For this review, take the finished solid that the model builds, in its own axes (mm). Give positions to 0.01 mm unless a question says otherwise; leave off trailing zeros. Write each loop counter-clockwise with the first axis right and the second up, starting at its lowest first coordinate (ties: lowest second). Pieces come first, ordered by that corner, then holes.
1) We need section A-A on x = 132. Give the boundary of the cut face in (y, z).
2) We need section C-C on y = 2.05. Give the boundary of the cut face in (x, z) (1 decimal), and give its area (3 significant figures).
3) We need section B-B on z = 356.5. Give the boundary of the cut face in (x, y), and give its area (3 significant figures).
4) Wall thickness on line 1 along Z through (x, y) = (-104, 2.1); line 2 along Z through (x, y) = (-29, 1.95): over which ranges is each line inside the solid? List them lowest first.
5) For P1, Ø1.5, axis at y = 1, z = 304.5, coming from the -X side, flat-tipped, find the tip position at first contact; note if it passes through.
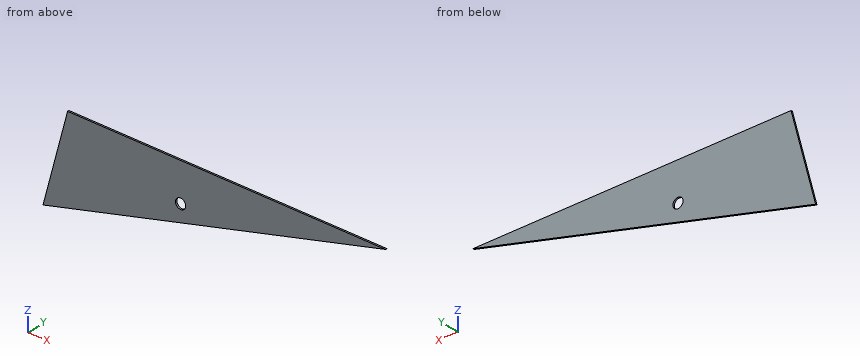
from build123d import *

# Parameters (mm, degrees)
BOSS_EXTRUDE1_DEPTH = 2.54
SKETCH2_R           = 7.9375
CUT_EXTRUDE1_DEPTH  = 2.54
CUT_EXTRUDE2_DEPTH  = 2.54


with BuildPart() as part:
    # Sketch1 → Boss-Extrude1 (new body)
    with BuildSketch(Plane(origin=(0, 0, 0), x_dir=(1, 0, 0), z_dir=(0, 1, 0))):
        Polygon((-288.635862607, -221.384099055), (-288.635862607, -365.420521122), (248.915382685, -365.420521122), align=None)
    extrude(amount=BOSS_EXTRUDE1_DEPTH)

    # Sketch2 → Cut-Extrude1 (cut)
    with BuildSketch(Plane(origin=(0, 2.54, 0), x_dir=(1, 0, 0), z_dir=(0, 1, 0))):
        with Locations((-72.735862607, -305.530344684)):
            Circle(SKETCH2_R)
    extrude(amount=-CUT_EXTRUDE1_DEPTH, mode=Mode.SUBTRACT)

    # Sketch3 → Cut-Extrude2 (cut)
    with BuildSketch(Plane.XZ):
        Polygon((-288.635862607, 221.384099055), (-250.041419634, 365.420521122), (-288.635862607, 365.420521122), align=None)
    extrude(amount=-CUT_EXTRUDE2_DEPTH, mode=Mode.SUBTRACT)


solid = part.part
Results list:
1. outline: (0, 334.09) - (2.54, 334.09) - (2.54, 365.42) - (0, 365.42) - close
2. outline: (-288.6, 221.4) - (248.9, 365.4) - (-250, 365.4) - close; hole circle Ø15.9 at (-72.7, 305.5)
2. area: 35,700 mm2
3. outline: (-252.43, 0) - (215.62, 0) - (215.62, 2.54) - (-252.43, 2.54) - close
3. area: 1,190 mm2
4. line 1: z = 270.86 to 365.42
4. line 2: z = 290.95 to 365.42
5. P1: stops at x = -266.57
